Build history of the part. All positions in model axes, mm. Face numbers are marked on the shaded views. A direction names the side the tool comes from. Round coordinates to 2 decimals unless told otherwise and drop trailing zeros. Write each loop counter-clockwise with the first axis right and the second up, starting at its lowest first coordinate (ties: lowest second). Pieces come first, ordered by that corner, then holes. Notation, with made-up numbers: (43, 76) -> (76, 76) arc R17 cw to (76, 84) -> close; hole circle Ø5 at (-9.75, 7). An arc over 180 degrees is marked (long way). Answer in a Markdown table with one row per item.
Autodesk Fusion 360 part; units mm, degrees
sketch "Esquisse1" plane through (0, 0, 0) normal (0, 0, 1) x (1, 0, 0)
  line L0 (0, 0) -> (73, 0)
  line L1 (73, 0) -> (73, 87)
  line L2 (73, 87) -> (-40, 87)
  line L3 (-40, 87) -> (-40, 17)
  line L4 (-40, 17) -> (0, 0)
  dimension "d5" = 87
  dimension "d6" = 113
  dimension "d7" = 70
  dimension "d8" = 73
extrude "Extrusion1" add sketch "Esquisse1" along normal blind 3
sketch "Esquisse2" plane through (0, 0, 3) normal (0, 0, 1) x (-1, 0, 0)
  line L0 (40, -17) -> (0, 0)
  line L1 (0, 0) -> (-73, 0)
  line L2 (-73, 0) -> (-73, -87)
  line L3 (-73, -87) -> (40, -87)
  line L4 (40, -87) -> (40, -17)
  line L5 (-0.8147, -4) -> (-69, -4)
  line L6 (-69, -4) -> (-69, -83)
  line L7 (-69, -83) -> (36, -83)
  line L8 (36, -83) -> (36, -19.6463)
  line L9 (36, -19.6463) -> (-0.8147, -4)
  dimension "d11" = 4
  dimension "d12" = 4
  dimension "d13" = 4
  dimension "d14" = 4
  dimension "d15" = 4
extrude "Extrusion2" add sketch "Esquisse2" along normal blind 15
sketch "Esquisse3" plane through (0, 0, 18) normal (0, 0, 1) x (-1, 0, 0)
  line L0 (-0.8147, -4) -> (36, -19.6463)
  line L1 (36, -19.6463) -> (36, -83)
  line L2 (36, -83) -> (-69, -83)
  line L3 (-69, -83) -> (-69, -4)
  line L4 (-69, -4) -> (-0.8147, -4)
  line L5 (40, -87) -> (40, -17)
  line L6 (40, -17) -> (0, 0)
  line L7 (0, 0) -> (-73, 0)
  line L8 (-73, 0) -> (-73, -87)
  line L9 (-73, -87) -> (40, -87)
  line L10 (37.6, -84.6) -> (-70.6, -84.6)
  line L11 (-70.6, -84.6) -> (-70.6, -2.4)
  line L12 (-70.6, -2.4) -> (-0.4888, -2.4)
  line L13 (-0.4888, -2.4) -> (37.6, -18.5878)
  line L14 (37.6, -18.5878) -> (37.6, -84.6)
  dimension "d18" = 1.6
  dimension "d19" = 1.6
  dimension "d20" = 1.6
  dimension "d21" = 1.6
  dimension "d22" = 1.6
extrude "Extrusion3" add sketch "Esquisse3" along normal blind 8 contours L10 L11 L12 L13 L14
sketch "Esquisse4" plane through (0, 0, 3) normal (0, 0, 1) x (-1, 0, 0)
  line L0 (-0.8147, -4) -> (-69, -4)
  line L1 (-69, -4) -> (-69, -83)
  line L2 (-69, -83) -> (36, -83)
  line L3 (36, -83) -> (36, -19.6463)
  line L4 (36, -19.6463) -> (-0.8147, -4)
  line L5 (-69, -83) -> (-10, -83)
  line L6 (-10, -83) -> (-10, -4)
  line L7 (-10, -4) -> (-69, -4)
  line L8 (-69, -4) -> (-69, -83)
  line L9 (36, -83) -> (-1.5, -83)
  line L10 (-1.5, -83) -> (-1.5, -19.6463)
  line L11 (-1.5, -19.6463) -> (36, -19.6463)
  line L12 (36, -19.6463) -> (36, -83)
  dimension "d25" = 59
  dimension "d27" = 37.5
extrude "Extrusion4" cut sketch "Esquisse4" against normal blind 1 contours L0 L1 L2 L5 L6 L7 L8 | L2 L3 L9 L10 L11 L12
sketch "Esquisse5" plane through (73, 0, 0) normal (1, 0, 0) x (0, 1, 0)
  line L0 (0, 0) -> (87, 0)
  line L1 (87, 0) -> (87, 18)
  line L2 (87, 18) -> (0, 18)
  line L3 (0, 18) -> (0, 0)
  line L4 (23, 14) -> (35, 14)
  arc A0 (35, 14) -> (35, 22) centre (35, 18) ccw
  line L5 (35, 22) -> (23, 22)
  arc A1 (23, 22) -> (23, 14) centre (23, 18) ccw
  line L6 (19, 18) -> (39, 18)
  line L7 (39, 18) -> (39, 26)
  line L8 (39, 26) -> (19, 26)
  line L9 (19, 26) -> (19, 18)
  line L10 (2.4, 26) -> (84.6, 26)
  dimension "d34" = 8
  dimension "d35" = 12
  dimension "d36" = 23
  dimension "d37" = 14
  dimension "d38" = 4
extrude "Extrusion5" cut sketch "Esquisse5" against normal blind 5 contours L2 A0 L5 A1 L6 | A0 L5 A1 L7 L8 L9 L10 | L2 L4 A0 A1 L6
sketch "Esquisse10" plane through (1.5646, 3.6813, 0) normal (0.3911, 0.9203, 0) x (-0.9203, 0.3911, 0)
  line L0 (0.8147, 3) -> (40.8164, 3)
  line L1 (40.8164, 3) -> (40.8164, 26)
  line L2 (40.8164, 26) -> (0.8147, 26)
  line L3 (0.8147, 26) -> (0.8147, 3)
  line L4 (3.8147, 26) -> (12.8147, 26)
  line L5 (12.8147, 26) -> (12.8147, 4)
  line L6 (12.8147, 4) -> (3.8147, 4)
  line L7 (3.8147, 4) -> (3.8147, 26)
  dimension "d55" = 9
  dimension "d56" = 22
  dimension "d57" = 3
extrude "Extrusion8" cut sketch "Esquisse10" along direction (-0.473316, -0.880893, 0) blind 5 contours L2 L4 L5 L6 L7
sketch "Esquisse11" plane through (0, 83, 0) normal (0, -1, 0) x (1, 0, 0)
  line L0 (69, 2) -> (69, 26)
  line L1 (69, 26) -> (-36, 26)
  line L2 (-36, 26) -> (-36, 2)
  line L3 (1.5, 2) -> (1.5, 3)
  line L4 (1.5, 3) -> (10, 3)
  line L5 (10, 3) -> (10, 2)
  line L6 (9.8, 26) -> (1.7, 26)
  line L7 (1.7, 26) -> (1.7, 6)
  line L8 (1.7, 6) -> (9.8, 6)
  line L9 (9.8, 6) -> (9.8, 26)
  line L10 (-36, 2) -> (1.5, 2)
  line L11 (10, 2) -> (69, 2)
  dimension "d60" = 8.1
  dimension "d61" = 20
  dimension "d62" = 0.2
extrude "Extrusion9" cut sketch "Esquisse11" against normal blind 5 contours L1 L6 L7 L8 L9
fillet "Congé1" radius 2 5 edges at (0, 0, 9) (73, 0, 9) (-40, 17, 9) (73, 87, 9) (-40, 87, 9)
fillet "Congé2" radius 1 2 edges at (-17.5926, 11.8231, 3) (5.4074, 4, 3)
fillet "Congé3" radius 1 3 edges at (73, 37.8284, 15.1716) (73, 29, 14) (73, 20.1716, 15.1716)
equation "d16 = 20 mm - 5 mm"
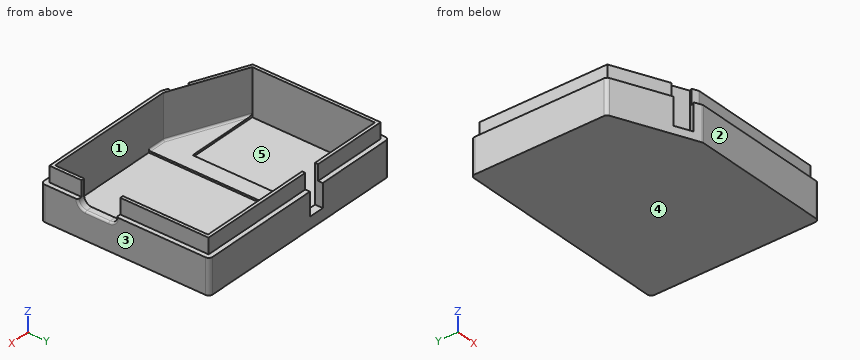
Q1. Saw through at B-B on x = 47.5. Write the cut outline in (y, z), plus the area to 3 significant figures.
A:
| item | result |
|---|---|
| outline | (0, 0) -> (87, 0) -> (87, 18) -> (84.6, 18) -> (84.6, 26) -> (83, 26) -> (83, 2) -> (4, 2) -> (4, 26) -> (2.4, 26) -> (2.4, 18) -> (0, 18) -> close |
| area | 328 mm² |
Q2. Saw through at C-C on z = 10. Write the cut outline in (x, y).
A:
| item | result |
|---|---|
| outline | (-40, 18.32) arc R2 ccw to (-38.78, 16.48) -> (-12.13, 5.16) -> (-10.23, 8.69) -> (-1.95, 5.17) -> (-3.85, 1.64) -> (-0.37, 0.16) arc R2 ccw to (0.41, 0) -> (71, 0) arc R2 ccw to (73, 2) -> (73, 85) arc R2 ccw to (71, 87) -> (9.8, 87) -> (9.8, 83) -> (69, 83) -> (69, 4) -> (0.81, 4) -> (-36, 19.65) -> (-36, 83) -> (1.7, 83) -> (1.7, 87) -> (-38, 87) arc R2 ccw to (-40, 85) -> close |
Q3. Which spindle directions (+Z, -Z, +X, -X, +Y, -Y) get a long thin tool onto all of the face, cutting with end or side? Do the marked faces 1 and 2. Say none if no direction does.
A:
| item | result |
|---|---|
| face 1 | +Z |
| face 2 | +Z, -Z, +X, -X, -Y |
Q4. Wall check: line 1 (X direction, y = 79, z = 23.5); line 2 (Y direction, x = 58.5, z = 23); line 3 (X direction, y = 52, z = 7.25). Give the ranges that are in metal, low to high. Write a range as [from, to].
A:
| item | result |
|---|---|
| line 1 | [-37.6, -36], [69, 70.6] |
| line 2 | [2.4, 4], [83, 84.6] |
| line 3 | [-40, -36], [69, 73] |
Q5. Two-plate mould, pull along X, no slides. Class the marked faces 3, 4 and 5: released by +X, released by -X, zero draft, split by the parting line, or undercut.
A:
| item | result |
|---|---|
| face 3 | released by +X |
| face 4 | zero draft |
| face 5 | undercut |
Q6. Saw through at D-D on y = 59.5. Write the cut outline in (x, z), plus the area to 3 significant figures.
A:
| item | result |
|---|---|
| outline | (-40, 0) -> (73, 0) -> (73, 18) -> (70.6, 18) -> (70.6, 26) -> (69, 26) -> (69, 2) -> (10, 2) -> (10, 3) -> (1.5, 3) -> (1.5, 2) -> (-36, 2) -> (-36, 26) -> (-37.6, 26) -> (-37.6, 18) -> (-40, 18) -> close |
| area | 388 mm² |
Q7. Saw through at A-A on z = 21. Write the cut outline in (x, y), plus the area to 3 significant figures.
A:
| item | result |
|---|---|
| outline | (-37.6, 18.59) -> (-10.99, 7.28) -> (-10.23, 8.69) -> (-1.95, 5.17) -> (-2.71, 3.76) -> (0.49, 2.4) -> (70.6, 2.4) -> (70.6, 19) -> (69, 19) -> (69, 4) -> (0.81, 4) -> (-36, 19.65) -> (-36, 83) -> (1.7, 83) -> (1.7, 84.6) -> (-37.6, 84.6) -> close; (9.8, 83) -> (69, 83) -> (69, 39) -> (70.6, 39) -> (70.6, 84.6) -> (9.8, 84.6) -> close |
| area | 519 mm² |
Q8. Drop flat-ended pins along their axis: P1, Ø9, axis at y = 11, z = 21, coming from the +X side; P2, Ø2.5, axis at y = 63, z = 23.5, coming from the -X side; P3, Ø6, axis at x = -12.5, z = 8.5, coming from the -Y side; P4, Ø6, axis at x = -2, y = 33.5, coming from the +Z side. Give the stop position or say it passes through.
A:
| item | result |
|---|---|
| P1 | x = 73 |
| P2 | x = -37.6 |
| P3 | y = 5.16 |
| P4 | z = 2 |
